The listing builds one solid part. Answer for the finished solid, in the listing's coordinates (mm). Face numbers are marked on the shaded views. A direction names the side the tool comes from. Coordinates: 2 decimals unless noted, no trailing zeros. Order: outer loops, then holes, each group sorted by start corner. A loop starts at its lowest first (then second) coordinate and runs counter-clockwise, first axis right, second up. Notation, with made-up numbers: (74.25, -2.75) - (118.25, -2.75) arc R23 ccw to (118.25, 8.25) - close; hole circle Ø8 at (80, -16.75). An arc over 180 degrees is marked (long way). Use a Markdown table: item, result. Add a question column.
Item 1: The part is cut by section B-B, the plane y = 0. State how many separate pieces and enclosed holes the cut face has, then the cut area to 3 significant figures.
Item 2: For the marked faces 1, 2 and 3, determine the directions among +Z, -Z, +X, -X, +Y, -Y from which every point of the face is accessible in a straight line to the end or side of a thin tool.
Item 3: Find the intervals of material crossed by line 1 along Z through (x, y) = (0.75, 3.5); line 2 along Z through (x, y) = (0, 0.5); line 3 along Z through (x, y) = (1, -0.5), in increasing order.
Item 4: The part is cut by section A-A, the plane z = 129. Give the vertices of the cut face in (x, y), then the cut area to 3 significant figures.
Item 5: Flat-ended cylindrical pins translate along their axes: P1, Ø2, axis at x = 0.5, z = 144, coming from the +Y side; P2, Ø1, axis at x = 2.5, z = 79, coming from the -Y side; P3, Ø0.5, axis at y = 3.5, z = 144, coming from the +X side. Find the tip coordinate at first contact, or state that the pin passes through.
Item 6: The part is cut by section C-C, the plane z = 144.5. Give the vertices of the cut face in (x, y).
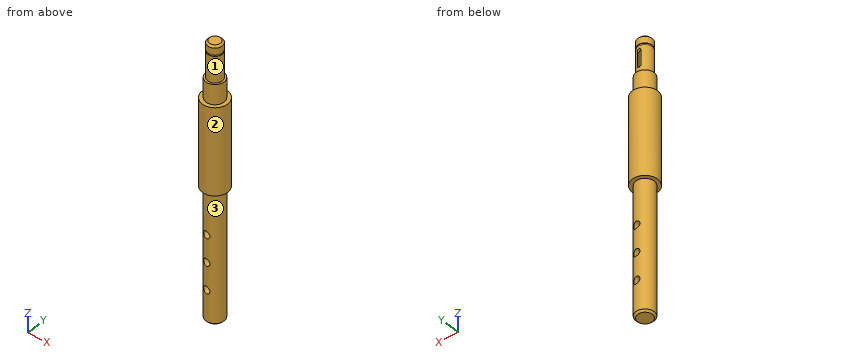
from build123d import *

# Parameters (mm, degrees)
SKETCH1_R           = 5
BOSS_EXTRUDE1_DEPTH = 136
SKETCH2_R           = 4
BOSS_EXTRUDE2_DEPTH = 20
CUT_EXTRUDE1_DEPTH  = 1.2
SKETCH4_W           = 0.55765723
SKETCH4_H           = 0.9
CHAMFER1_SIZE       = 1
SKETCH6_R           = 7
BOSS_EXTRUDE3_DEPTH = 48
CUT_EXTRUDE3_REACH  = 159.949
SKETCH7_R           = 2
SKETCH8_R           = 5
CUT_EXTRUDE4_DEPTH  = 5
CHAMFER2_SIZE       = 1


with BuildPart() as part:
    # Sketch1 → Boss-Extrude1 (new body)
    with BuildSketch(Plane.XY):
        Circle(SKETCH1_R)
    extrude(amount=BOSS_EXTRUDE1_DEPTH)

    # Sketch2 → Boss-Extrude2 (add)
    with BuildSketch(Plane.XY.offset(136)):
        Circle(SKETCH2_R)
    extrude(amount=BOSS_EXTRUDE2_DEPTH)

    # Sketch3 → Cut-Extrude1 (cut)
    with BuildSketch(Plane(origin=(0, 4, 0), x_dir=(1, 0, 0), z_dir=(0, 1, 0))):
        with BuildLine():
            Line((-1, -148), (-1, -140))
            ThreePointArc((-1, -140), (0, -139), (1, -140))
            Line((1, -140), (1, -148))
            ThreePointArc((1, -148), (0, -149), (-1, -148))
        make_face()
    extrude(amount=-CUT_EXTRUDE1_DEPTH, mode=Mode.SUBTRACT)

    # Sketch4 → Cut-Revolve1 (revolve, cut)
    with BuildSketch(Plane(origin=(0, 0, 0), x_dir=(1, 0, 0), z_dir=(0, 1, 0))):
        with Locations((-4.078828615, -150.95)):
            Rectangle(SKETCH4_W, SKETCH4_H)
    revolve(axis=Axis((0, 0, -16.531983683), (0, 0, 1)), mode=Mode.SUBTRACT)

    # Chamfer1
    chamfer1_edges = [part.edges().sort_by_distance(p)[0] for p in [
        (-4, 0, 156),
    ]]
    chamfer(chamfer1_edges, length=CHAMFER1_SIZE)

    # Sketch6 → Boss-Extrude3 (add)
    with BuildSketch(Plane.XY.offset(77)):
        Circle(SKETCH6_R)
    extrude(amount=BOSS_EXTRUDE3_DEPTH)

    # Sketch7 → Cut-Extrude3 (cut, up to next)
    with BuildSketch(Plane(origin=(-2.642522108, -15.780274931, 0), x_dir=(0, 0, 1), z_dir=(-0.16515763172219566, -0.9862671832135123, -1.0705486064346984e-15)), mode=Mode.PRIVATE) as cut_extrude3_sk1:
        with Locations(Location((53, 0, 0), (0, 0, 270))):
            Circle(SKETCH7_R)
    cut_extrude3_tool1 = extrude(cut_extrude3_sk1.sketch, amount=-CUT_EXTRUDE3_REACH, mode=Mode.PRIVATE) & part.part
    # Sketch7 → Cut-Extrude3 (cut, up to next)
    with BuildSketch(Plane(origin=(-2.642522108, -15.780274931, 0), x_dir=(0, 0, 1), z_dir=(-0.16515763172219566, -0.9862671832135123, -1.0705486064346984e-15)), mode=Mode.PRIVATE) as cut_extrude3_sk2:
        with Locations(Location((38, 0, 0), (0, 0, 270))):
            Circle(SKETCH7_R)
    cut_extrude3_tool2 = extrude(cut_extrude3_sk2.sketch, amount=-CUT_EXTRUDE3_REACH, mode=Mode.PRIVATE) & part.part
    # Sketch7 → Cut-Extrude3 (cut, up to next)
    with BuildSketch(Plane(origin=(-2.642522108, -15.780274931, 0), x_dir=(0, 0, 1), z_dir=(-0.16515763172219566, -0.9862671832135123, -1.0705486064346984e-15)), mode=Mode.PRIVATE) as cut_extrude3_sk3:
        with Locations(Location((23, 0, 0), (0, 0, 270))):
            Circle(SKETCH7_R)
    cut_extrude3_tool3 = extrude(cut_extrude3_sk3.sketch, amount=-CUT_EXTRUDE3_REACH, mode=Mode.PRIVATE) & part.part
    add(cut_extrude3_tool1.solids().sort_by_distance((-2.642522, -15.780275, 53))[0], mode=Mode.SUBTRACT)
    add(cut_extrude3_tool2.solids().sort_by_distance((-2.642522, -15.780275, 38))[0], mode=Mode.SUBTRACT)
    add(cut_extrude3_tool3.solids().sort_by_distance((-2.642522, -15.780275, 23))[0], mode=Mode.SUBTRACT)

    # Sketch8 → Cut-Extrude4 (cut)
    with BuildSketch(Plane(origin=(0, 0, 0), x_dir=(-1, 0, 0), z_dir=(0, 0, -1))):
        Circle(SKETCH8_R)
    extrude(amount=-CUT_EXTRUDE4_DEPTH, mode=Mode.SUBTRACT)

    # Chamfer2
    chamfer2_edges = [part.edges().sort_by_distance(p)[0] for p in [
        (-5, 0, 5),
    ]]
    chamfer(chamfer2_edges, length=CHAMFER2_SIZE)


solid = part.part
Solution:
| question | item | result |
|---|---|---|
| 1 | separate pieces | 1 |
| 1 | enclosed holes | 3 |
| 1 | area | 1,620 mm2 |
| 2 | face 1 | +Z |
| 2 | face 2 | +Z, -Z |
| 2 | face 3 | -Z |
| 3 | line 1 | z = 5 to 21.01, 24.99 to 36.01, 39.99 to 51.01, 54.99 to 139.34, 148.66 to 155.42 |
| 3 | line 2 | z = 5 to 21, 25 to 36, 40 to 51, 55 to 156 |
| 3 | line 3 | z = 5 to 21.31, 24.69 to 36.31, 39.69 to 51.31, 54.69 to 156 |
| 4 | outline | circle Ø10 at (0, 0) |
| 4 | area | 78.5 mm2 |
| 5 | P1 | stops at y = 3.87 |
| 5 | P2 | stops at y = -6.71 |
| 5 | P3 | stops at x = 2.33 |
| 6 | outline | (-1, 2.8) - (-1, 3.87) arc R4 ccw (long way) to (1, 3.87) - (1, 2.8) - close |
